Source: CAD feature listing. Evaluate the final solid. Frame: model axes, mm. A direction names the side the tool comes from. Give positions to 0.01 mm unless a question says otherwise; leave off trailing zeros. Order: outer loops, then holes, each group sorted by start corner. A loop starts at its lowest first (then second) coordinate and runs counter-clockwise, first axis right, second up. Notation, with made-up numbers: M 59.5,-7 L 116.5,-7 A19 ccw 116.5,6 Z; hole C -4.75,-17 d2. An arc over 180 degrees is marked long. Answer as a JSON object with one key per item and string values. Group by question number.
1. Material intervals for L1, parallel to Y at x = 14, z = -12; L2, parallel to Z at x = 11, y = -22; L3, parallel to Z at x = 43.5, y = 6, sorted ascending. Write a range as [from, to].
2. Pin query (flat end, axial travel): P1, Ø21, axis at x = 36.5, y = 4.5, coming from the -Z side; P2, Ø1.6, axis at x = 25, y = 21, coming from the -Z side; P3, Ø6.5, axis at x = 13, z = -8.5, coming from the -Y side. Return the tip coordinate at first contact, or that it passes through.
3. Section query B-B (x = 17.5). Output: boundary loops of the cut face in (y, z).
4. Set-up query: faces 1 (the flat face through (25, 21, -12.293)), 2 (the flat face through (25, -21, -6)), 3 (the flat face through (5, -1, -8)), 4 (the flat face through (12, -6.21, -8)), 5 (the flat face through (20, -1, -8)). Return all of +Z, -Z, +X, -X, +Y, -Y with unobstructed straight access to the full face (end or side cutting, diameter ignored); none if empty.
5. Section query D-D (y = -30). Output: boundary loops of the cut face in (x, z), plus the area to 3 significant figures.
6. Section query C-C (z = -13.5). Output: boundary loops of the cut face in (x, y), plus the area to 3 significant figures.
7. Section query A-A (x = 37). Output: boundary loops of the cut face in (y, z), plus the area to 4 significant figures.
8. Pull-direction query (Y, two-part tool) for faces 6 (the flat face through (25, -13.71, -5)), 7 (the flat face through (25, 33.29, 1)), 8 (the flat face through (25, -28.71, -5)); classes: +Y half, -Y half, draft (parallel to the pull), parting line (faces both ways), or undercut.
from build123d import *

# Parameters (mm, degrees)
F0_R     = 3.5
F1_DEPTH = 50
F2_SIZE  = 1
F3_W     = 30
F3_H     = 8
F3_W_2   = 5
F4_DEPTH = 10


with BuildPart() as f1:
    # F0 (on Right) → F1 (new body)
    with BuildSketch(Plane.YZ):
        with BuildLine():
            Line((33.2899148837, -4), (33.2899148837, 6))
            Line((33.2899148837, 6), (-33.7100851163, 6))
            Line((-33.7100851163, 6), (-33.7100851163, -4))
            Line((-33.7100851163, -4), (-28.7100851163, -4))
            Line((-28.7100851163, -4), (-28.7100851163, -6))
            Line((-28.7100851163, -6), (-13.7100851163, -6))
            Line((-13.7100851163, -6), (-13.7100851163, -4))
            Line((-13.7100851163, -4), (-6.2100851163, -4))
            Line((-6.2100851163, -4), (-6.2100851163, -12))
            ThreePointArc((-6.2100851163, -12), (-1.2100851163, -17), (3.7899148837, -12))
            Line((3.7899148837, -12), (3.7899148837, -4))
            Line((3.7899148837, -4), (12.2899148837, -4))
            Line((12.2899148837, -4), (21.2899148837, -13))
            Line((21.2899148837, -13), (30.2899148837, -4))
            Line((30.2899148837, -4), (33.2899148837, -4))
        make_face()
        with Locations((-1.2100851163, -12)):
            Circle(F0_R, mode=Mode.SUBTRACT)
    extrude(amount=F1_DEPTH)

    # F2
    f2_edges = [f1.edges().sort_by_distance(p)[0] for p in [
        (25, 21.289915, -13),
    ]]
    chamfer(f2_edges, length=F2_SIZE)

    # F3 (on face) → F4 (cut, through all)
    with BuildSketch(Plane.XZ.offset(6.2100851163)):
        with Locations((35, -8)):
            Rectangle(F3_W, F3_H)
        Polygon((79.836667031, -4), (50, -4), (50, -12), (20, -12), (20, -31.4453998581), (79.836667031, -31.4453998581), align=None)
        with Locations((2.5, -8)):
            Rectangle(F3_W_2, F3_H)
        Polygon((5, -31.5237529576), (5, -12), (0, -12), (0, -4), (-35.2658848278, -4), (-35.2658848278, -31.5237529576), align=None)
    extrude(amount=-F4_DEPTH, mode=Mode.SUBTRACT)


solid = f1.part
Answer sheet:
{
 "1": {"L1": "[-6.21, -4.71], [2.29, 3.79], [20.29, 22.29]", "L2": "[-6, 6]", "L3": "[-4, 6]"},
 "2": {"P1": "z = -6.71", "P2": "z = -12.29", "P3": "y = -28.71"},
 "3": {"outline": "M -33.71,-4 L -28.71,-4 L -28.71,-6 L -13.71,-6 L -13.71,-4 L -6.21,-4 L -6.21,-12 A5 ccw 3.79,-12 L 3.79,-4 L 12.29,-4 L 20.58,-12.29 L 22,-12.29 L 30.29,-4 L 33.29,-4 L 33.29,6 L -33.71,6 Z; hole C -1.21,-12 d7"},
 "4": {"face 1": "-Z, +X, -X, +Y", "face 2": "-Z, +X, -X, -Y", "face 3": "-Z, -X", "face 4": "-Z, +X, -X", "face 5": "-Z, +X"},
 "5": {"outline": "M 0,-4 L 50,-4 L 50,6 L 0,6 Z", "area": "500 mm^2"},
 "6": {"outline": "M 5,-5.98 L 20,-5.98 L 20,-4.37 L 5,-4.37 Z; M 5,1.95 L 20,1.95 L 20,3.56 L 5,3.56 Z", "area": "48.2 mm^2"},
 "7": {"outline": "M -33.71,-4 L -28.71,-4 L -28.71,-6 L -13.71,-6 L -13.71,-4 L 12.29,-4 L 20.58,-12.29 L 22,-12.29 L 30.29,-4 L 33.29,-4 L 33.29,6 L -33.71,6 Z", "area": "780.5 mm^2"},
 "8": {"face 6": "undercut", "face 7": "+Y half", "face 8": "-Y half"}
}
